CAD build for the part. Positions are in the model's coordinates, mm. Round coordinates to 2 decimals unless told otherwise and drop trailing zeros. Write each loop counter-clockwise with the first axis right and the second up, starting at its lowest first coordinate (ties: lowest second). Pieces come first, ordered by that corner, then holes. Notation, with made-up numbers: (33.5, 33) - (88.5, 33) arc R34 ccw to (88.5, 65) - close; hole circle Ø3 at (-1, 7.5). An arc over 180 degrees is marked (long way). Put each result on its own line as item: value. Start each with the question number.
Item 1: Cut at D-D (x = 5). Give the cut face in (y, z), and give its area (3 significant figures).
Item 2: Pin check, flat tips, straight feed: pin 1 Ø6 at (x, z) = (-5, -12) entering from +Y; pin 2 Ø1 at (y, z) = (2.5, -14.5) entering from +X. Stop position of each tip, or through.
Item 3: Mould opens along Y. For faces 1 (the cylindrical face through (-0.69, -3.1, -12.52)), 2 (the flat face through (-3, -16, -13)), 3 (the flat face through (-2, -5, 0)) say: released by +Y, released by -Y, zero draft, split by the parting line, or undercut.
Item 4: Drill centre lines: line 1 (Y direction, x = 0, z = -15.75) (3 decimals); line 2 (Y direction, x = -1.25, z = -5); line 3 (X direction, y = 1, z = -11.75). Where is each one in solid material? Low to high. Write a range as from..to.
Item 5: Cut at A-A (x = -2.25). Give the cut face in (y, z), and give its area (3 significant figures).
Item 6: Cut at C-C (z = -3.25). Give the cut face in (x, y) (3 decimals).
Item 7: Cut at B-B (y = -0.75). Give the cut face in (x, z), and give its area (3 significant figures).
Autodesk Inventor part; units mm, degrees
ref_plane "YZ Plane" through (0, 0, 0) normal (1, 0, 0) x (0, 1, 0)
ref_plane "XZ Plane" through (0, 0, 0) normal (0, 1, 0) x (-1, 0, 0)
ref_plane "XY Plane" through (0, 0, 0) normal (0, 0, 1) x (1, 0, 0)
sketch "Sketch1" plane through (0, 0, 0) normal (0, 0, 1) x (1, 0, 0)
  circle A0 centre (0, 0) radius 3.175
  circle A1 centre (0, 0) radius 6.35
  line L0 (-0.35, -16) -> (-6.35, -16)
  line L1 (-6.35, -16) -> (-6.35, 0)
  line L2 (-0.35, -16) -> (5.7723, -2.6464)
  dimension "d0" = 6.35
  dimension "d1" = 12.7
  dimension "d29" = 6
extrude "Extrusion1" add sketch "Sketch1" against normal blind 25.4
properties part number "Servo Mount"
Output values:
1. outline: (-4.33, -25.4) - (3.91, -25.4) - (3.91, 0) - (-4.33, 0) - close
1. area: 209 mm2
2. pin 1: y = 6.03
2. pin 2: x = 6.03
3. face 1: undercut
3. face 2: released by -Y
3. face 3: zero draft
4. line 1: -15.237..-3.175, 3.175..6.35
4. line 2: -16..-2.92, 2.92..6.23
4. line 3: -6.27..-3.01, 3.01..6.27
5. outline: (-16, -25.4) - (-2.24, -25.4) - (-2.24, 0) - (-16, 0) - close; (2.24, -25.4) - (5.94, -25.4) - (5.94, 0) - (2.24, 0) - close
5. area: 443 mm2
6. outline: (-6.35, -16) - (-0.35, -16) - (5.772, -2.646) arc R6.35 ccw (long way) to (-6.35, 0) - close; hole circle Ø6.35 at (0, 0)
7. outline: (-6.35, -25.4) - (-3.09, -25.4) - (-3.09, 0) - (-6.35, 0) - close; (3.09, -25.4) - (6.31, -25.4) - (6.31, 0) - (3.09, 0) - close
7. area: 165 mm2
